Could you check a few things on this model? Use its own coordinates, in mm. A direction names the side the tool comes from. Round coordinates to 2 decimals unless told otherwise and drop trailing zeros. Loops run counter-clockwise (first coordinate to the right, second up) from the corner with the lowest first, then second, coordinate; pieces in that order, holes last.
from build123d import *

# Parameters (mm, degrees)
ESQUISSE1_W      = 30.8
ESQUISSE1_H      = 12.5
ESQUISSE1_R      = 1.847277142
ESQUISSE1_R_2    = 1.96687405
EXTRUSION1_DEPTH = 1
EXTRUSION2_DEPTH = 6
ESQUISSE3_W      = 19.2
ESQUISSE3_H      = 10
EXTRUSION3_DEPTH = 6
ESQUISSE4_R      = 0.272537765
EXTRUSION4_DEPTH = 4.8
CONG_1_R         = 1
EXTRUSION5_START = 6
ESQUISSE7_R      = 0.272537765
EXTRUSION5_DEPTH = 6


with BuildPart() as part:
    # Esquisse1 → Extrusion1 (new body)
    with BuildSketch(Plane.XY):
        with Locations((15.4, 6.25)):
            Rectangle(ESQUISSE1_W, ESQUISSE1_H)
        with Locations((2.9, 6.25)):
            Circle(ESQUISSE1_R, mode=Mode.SUBTRACT)
        with Locations((27.9, 6.25)):
            Circle(ESQUISSE1_R_2, mode=Mode.SUBTRACT)
    extrude(amount=EXTRUSION1_DEPTH)

    # Esquisse2 → Extrusion2 (add)
    with BuildSketch(Plane.XY.offset(1)):
        with BuildLine():
            Line((8.441753593, 10.569106944), (22.358246407, 10.569106944))
            ThreePointArc((22.358246407, 10.569106944), (23.124290851, 10.211894554), (23.34305416, 9.395458766))
            Line((23.34305416, 9.395458766), (22.302724974, 3.495458766))
            ThreePointArc((22.302724974, 3.495458766), (21.960704831, 2.903062501), (21.317917221, 2.669106944))
            Line((21.317917221, 2.669106944), (9.482082779, 2.669106944))
            ThreePointArc((9.482082779, 2.669106944), (8.839295169, 2.903062501), (8.497275026, 3.495458766))
            Line((8.497275026, 3.495458766), (7.45694584, 9.395458766))
            ThreePointArc((7.45694584, 9.395458766), (7.675709149, 10.211894554), (8.441753593, 10.569106944))
        make_face()
    extrude(amount=EXTRUSION2_DEPTH)

    # Esquisse3 → Extrusion3 (add)
    with BuildSketch(Plane(origin=(0, 0, 0), x_dir=(-1, 0, 0), z_dir=(0, 0, -1))):
        with Locations((-15.4, 6.25)):
            Rectangle(ESQUISSE3_W, ESQUISSE3_H)
    extrude(amount=EXTRUSION3_DEPTH)

    # Esquisse4 → Extrusion4 (add)
    with BuildSketch(Plane(origin=(0, 0, -6), x_dir=(-1, 0, 0), z_dir=(0, 0, -1))):
        with Locations((-19.98, 8.23)):
            Circle(ESQUISSE4_R)
        with Locations((-17.69, 8.23)):
            Circle(ESQUISSE4_R)
        with Locations((-15.4, 8.23)):
            Circle(ESQUISSE4_R)
        with Locations((-13.11, 8.23)):
            Circle(ESQUISSE4_R)
        with Locations((-10.82, 8.23)):
            Circle(ESQUISSE4_R)
        with Locations((-9.68, 6.25)):
            Circle(ESQUISSE4_R)
        with Locations((-11.97, 6.25)):
            Circle(ESQUISSE4_R)
        with Locations((-14.149725584, 6.068095869)):
            Circle(ESQUISSE4_R)
        with Locations((-16.529732269, 6.22882427)):
            Circle(ESQUISSE4_R)
        with Locations((-18.84, 6.25)):
            Circle(ESQUISSE4_R)
        with Locations((-19.98, 4.27)):
            Circle(ESQUISSE4_R)
        with Locations((-17.69, 4.27)):
            Circle(ESQUISSE4_R)
        with Locations((-15.4, 4.27)):
            Circle(ESQUISSE4_R)
        with Locations((-13.11, 4.27)):
            Circle(ESQUISSE4_R)
        with Locations((-10.82, 4.27)):
            Circle(ESQUISSE4_R)
    extrude(amount=EXTRUSION4_DEPTH)

    # Congé1
    cong_1_edges = [part.edges().sort_by_distance(p)[0] for p in [
        (25, 11.25, -3),
        (25, 1.25, -3),
        (5.8, 1.25, -3),
        (5.8, 11.25, -3),
        (25, 6.25, -6),
        (15.4, 1.25, -6),
        (5.8, 6.25, -6),
        (15.4, 11.25, -6),
        (0, 12.5, 0.5),
        (30.8, 12.5, 0.5),
        (30.8, 0, 0.5),
        (0, 0, 0.5),
    ]]
    fillet(cong_1_edges, radius=CONG_1_R)

    # Esquisse7 → Extrusion5 (cut)
    with BuildSketch(Plane.XY.offset(1).offset(EXTRUSION5_START)):
        with Locations(Location((19.98, 8.23, 0), (0, 0, 180))):
            Circle(ESQUISSE7_R)
        with Locations(Location((17.69, 8.23, 0), (0, 0, 180))):
            Circle(ESQUISSE7_R)
        with Locations(Location((15.4, 8.23, 0), (0, 0, 180))):
            Circle(ESQUISSE7_R)
        with Locations(Location((13.11, 8.23, 0), (0, 0, 180))):
            Circle(ESQUISSE7_R)
        with Locations(Location((10.82, 8.23, 0), (0, 0, 180))):
            Circle(ESQUISSE7_R)
        with Locations(Location((9.68, 6.25, 0), (0, 0, 180))):
            Circle(ESQUISSE7_R)
        with Locations(Location((11.97, 6.25, 0), (0, 0, 180))):
            Circle(ESQUISSE7_R)
        with Locations(Location((14.149725584, 6.068095869, 0), (0, 0, 180))):
            Circle(ESQUISSE7_R)
        with Locations(Location((16.529732269, 6.22882427, 0), (0, 0, 180))):
            Circle(ESQUISSE7_R)
        with Locations(Location((18.84, 6.25, 0), (0, 0, 180))):
            Circle(ESQUISSE7_R)
        with Locations(Location((19.98, 4.27, 0), (0, 0, 180))):
            Circle(ESQUISSE7_R)
        with Locations(Location((17.69, 4.27, 0), (0, 0, 180))):
            Circle(ESQUISSE7_R)
        with Locations(Location((15.4, 4.27, 0), (0, 0, 180))):
            Circle(ESQUISSE7_R)
        with Locations(Location((13.11, 4.27, 0), (0, 0, 180))):
            Circle(ESQUISSE7_R)
        with Locations(Location((10.82, 4.27, 0), (0, 0, 180))):
            Circle(ESQUISSE7_R)
    extrude(amount=-EXTRUSION5_DEPTH, mode=Mode.SUBTRACT)


solid = part.part
Item 1: We'd pull the mould along Y, two halves only. Please class faces 1 (the cylindrical face through (15.28, 10.965, -5.699)), 2 (the flat face through (0, 6.2, 0.5)), 3 (the cylindrical face through (26.45, 7.58, 0.49)): released by +Y, released by -Y, zero draft, split by the parting line, or undercut.
Results list:
face 1: released by +Y
face 2: zero draft
face 3: undercut
Item 2: If we section it at B-B, the plane z = -4: Please give me the cut outline in (x, y), then the cut area to 3 significant figures.
Results list:
outline: (5.8, 2.25) arc R1 ccw to (6.8, 1.25) - (24, 1.25) arc R1 ccw to (25, 2.25) - (25, 10.25) arc R1 ccw to (24, 11.25) - (6.8, 11.25) arc R1 ccw to (5.8, 10.25) - close
area: 191 mm2
Item 3: Will these pins go through, and if not, where does the flat tip stop? pin 1 (4 mm diameter, centred on x = 19, y = 7, fed in from -Z); pin 2 (1.5 mm diameter, centred on x = 10, z = -1, fed in from +Y); pin 3 (4 mm diameter, centred on x = 15, z = -2.5, fed in from -Y); pin 4 (2 mm diameter, centred on y = 8.5, z = -4, fed in from -X).
Results list:
pin 1: stops at z = -10.8
pin 2: stops at y = 11.25
pin 3: stops at y = 1.25
pin 4: stops at x = 5.8
Item 4: If we section it at A-A, the plane x = 2.9: Please give me the cut outline in (y, z).
Results list:
outline: (0, 0) - (4.4, 0) - (4.4, 1) - (0, 1) - close; (8.1, 0) - (12.5, 0) - (12.5, 1) - (8.1, 1) - close
Item 5: If we section it at C-C, the plane y = 5: Please give me the cut outline in (x, z).
Results list:
outline: (0, 0) - (1.54, 0) - (1.54, 1) - (0, 1) - close; (4.26, 0) - (5.8, 0) - (5.8, -5) arc R1 ccw to (6.8, -6) - (24, -6) arc R1 ccw to (25, -5) - (25, 0) - (26.38, 0) - (26.38, 1) - (22.57, 1) - (22.57, 7) - (8.23, 7) - (8.23, 1) - (4.26, 1) - close; (29.42, 0) - (30.8, 0) - (30.8, 1) - (29.42, 1) - close
Item 6: If I drill on line 1 along Y through (x, z) = (19.98, 2.8); line 2 along Y through (x, z) = (27.9, 0.6); line 3 along Y through (x, z) = (11.97, 2.6), over which ranges is the centre line in solid material (lowest first)?
Results list:
line 1: y = 2.67 to 4, 4.54 to 7.96, 8.5 to 10.57
line 2: y = 0 to 4.28, 8.22 to 12.5
line 3: y = 2.67 to 5.98, 6.52 to 10.57
Item 7: If we section it at D-D, the plane z = -8.75: Count the separate pieces of the cut face and the enclosed holes in it, then the cut area to 3 significant figures.
Results list:
separate pieces: 15
enclosed holes: 0
area: 3.50 mm2
Item 8: For faces 4 (the flat face through (22.83, 6.49, 3.96)), 5 (the flat face through (25, 6, -2)), 6 (the cylindrical face through (24.715, 1.551, -2.535)), which set-ups out of +Z, -Z, +X, -X, +Y, -Y let a thin tool reach every point of the face, with its end or its side?
Results list:
face 4: +Z, +X, -Y
face 5: -Z, +X, +Y, -Y
face 6: -Z, +X, -Y
